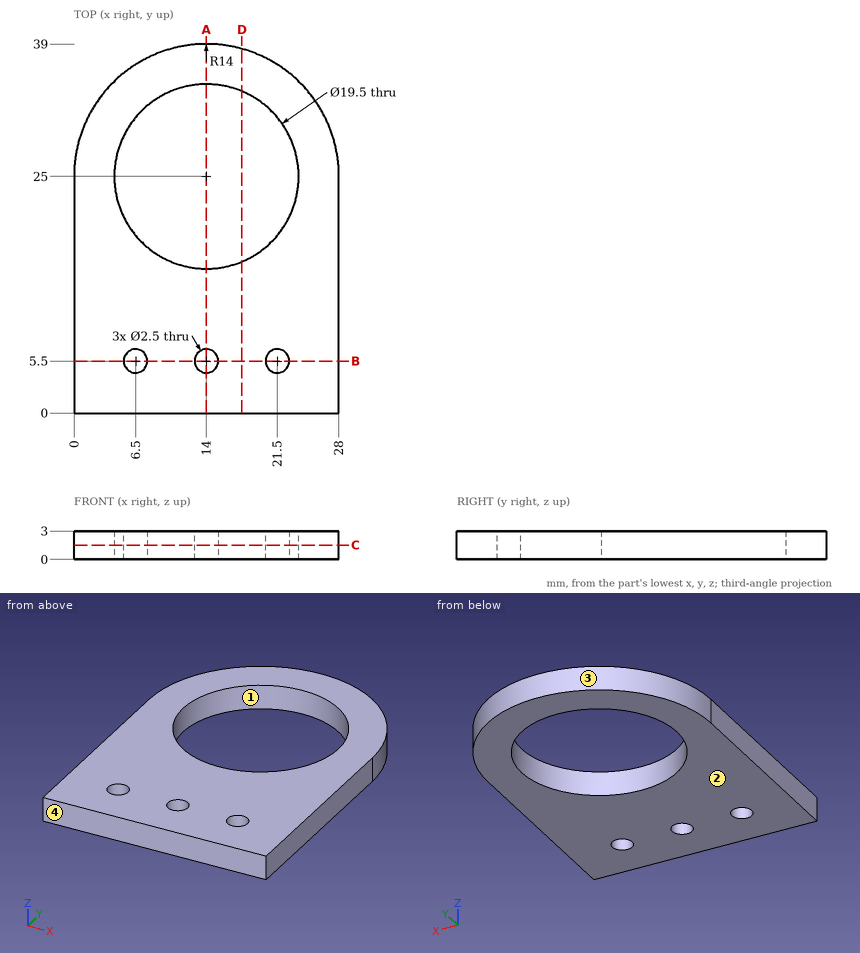
Geometry check sheet. Reference: drawing and pictorial views, mm from the part's lowest x, y, z. Round coordinates to 2 decimals unless told otherwise and drop trailing zeros. Loops run counter-clockwise (first coordinate to the right, second up) from the corner with the lowest first, then second, coordinate; pieces in that order, holes last.
1. Mould release check, pull along Y, two halves, no side actions. Record for the marked faces 1, 2, 3 and 4: released by +Y, released by -Y, zero draft, split by the parting line, or undercut.
2. Scan lines: probe 1 along Y at (x, z) = (14, 1.2); probe 2 along Y at (x, z) = (21.5, 1.8); probe 3 along Y at (x, z) = (20, 0.9). Record each from-to range of solid material in increasing order.
3. Sectioned sample at B-B on y = 5.5. Record the boundary of the cut face in (x, z), and give its area (3 significant figures).
4. Sectioned sample at A-A on x = 14. Record the boundary of the cut face in (y, z), and give its area (3 significant figures).
5. Sectioned sample at C-C on z = 1.5. Record the boundary of the cut face in (x, y).
6. Sectioned sample at D-D on x = 17.75. Record the boundary of the cut face in (y, z), and give its area (3 significant figures).
7. Gauge pin test, flat end, axial feed: pin 1 Ø1.5 at (x, y) = (21.5, 5.5) entering from +Z. Record the tip position at first contact, or that the pin passes through.
Recorded:
1. face 1: undercut
1. face 2: zero draft
1. face 3: released by +Y
1. face 4: released by -Y
2. probe 1: y = 0 to 4.25, 6.75 to 15.25, 34.75 to 39
2. probe 2: y = 0 to 4.25, 6.75 to 18.77, 31.23 to 36.82
2. probe 3: y = 0 to 17.31, 32.69 to 37.65
3. outline: (0, 0) - (5.25, 0) - (5.25, 3) - (0, 3) - close; (7.75, 0) - (12.75, 0) - (12.75, 3) - (7.75, 3) - close; (15.25, 0) - (20.25, 0) - (20.25, 3) - (15.25, 3) - close; (22.75, 0) - (28, 0) - (28, 3) - (22.75, 3) - close
3. area: 61.5 mm2
4. outline: (0, 0) - (4.25, 0) - (4.25, 3) - (0, 3) - close; (6.75, 0) - (15.25, 0) - (15.25, 3) - (6.75, 3) - close; (34.75, 0) - (39, 0) - (39, 3) - (34.75, 3) - close
4. area: 51.0 mm2
5. outline: (0, 0) - (28, 0) - (28, 25) arc R14 ccw to (0, 25) - close; hole circle Ø19.5 at (14, 25); hole circle Ø2.5 at (6.5, 5.5); hole circle Ø2.5 at (14, 5.5); hole circle Ø2.5 at (21.5, 5.5)
6. outline: (0, 0) - (16, 0) - (16, 3) - (0, 3) - close; (34, 0) - (38.49, 0) - (38.49, 3) - (34, 3) - close
6. area: 61.5 mm2
7. pin 1: passes through
